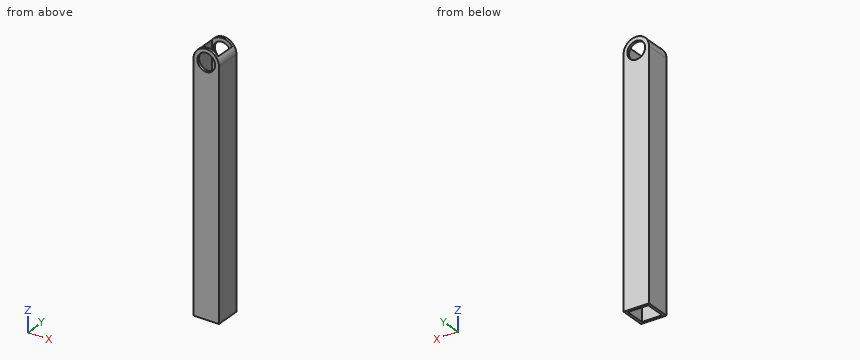
from build123d import *

# Parameters (mm, degrees)
SKETCH_1_W          = 10
SKETCH_1_H          = 10
SKETCH_1_W_2        = 8
SKETCH_1_H_2        = 8
EXTRUDE_1_DEPTH     = 100
SKETCH_2_R          = 3.5
CUT_EXTRUDE_1_DEPTH = 100


with BuildPart() as part:
    # ｽｹｯﾁ1 → ﾎﾞｽ - 押し出し1 (new body)
    with BuildSketch(Plane.XY):
        Rectangle(SKETCH_1_W, SKETCH_1_H)
        Rectangle(SKETCH_1_W_2, SKETCH_1_H_2, mode=Mode.SUBTRACT)
    extrude(amount=EXTRUDE_1_DEPTH)

    # ｽｹｯﾁ2 → ｶｯﾄ - 押し出し1 (cut)
    with BuildSketch(Plane(origin=(0, 5, 0), x_dir=(1, 0, 0), z_dir=(0, 1, 0))):
        with Locations(Location((0, -95, 0), (0, 0, 270))):
            Circle(SKETCH_2_R)
        with BuildLine():
            Line((-5, -95), (-5, -103))
            Line((-5, -103), (5, -103))
            Line((5, -103), (5, -95))
            ThreePointArc((5, -95), (0, -100), (-5, -95))
        make_face()
    extrude(amount=-CUT_EXTRUDE_1_DEPTH, mode=Mode.SUBTRACT)


solid = part.part
Could you check a few things on this model? Use its own coordinates, in mm. Round coordinates to 2 decimals unless told otherwise and drop trailing zeros. Write each loop counter-clockwise with the first axis right and the second up, starting at its lowest first coordinate (ties: lowest second). Pieces come first, ordered by that corner, then holes. Notation, with made-up numbers: (54, 74.25) - (98, 74.25) arc R31 cw to (98, 103.25) - close; hole circle Ø3 at (-35, 63.25). An arc over 180 degrees is marked (long way). Use a Markdown table: item, result.
Q1. I want a section at B-B (y = 2). List the corners of the cut face in (x, z) for me, plus the area to 3 significant figures.
Output values:
| item | result |
|---|---|
| outline | (-5, 0) - (-4, 0) - (-4, 98) arc R5 ccw to (-5, 95) - close; (4, 0) - (5, 0) - (5, 95) arc R5 ccw to (4, 98) - close |
| area | 194 mm2 |
Q2. For pin 1 (1 mm diameter, centred on x = -2, y = -0.5, fed in from +Z), with a flat end and sliding along its axis, tell me the tip position at first contact or that it passes through.
Output values:
| item | result |
|---|---|
| pin 1 | through |
Q3. I want a section at C-C (x = 1.75). List the corners of the cut face in (y, z) for me.
Output values:
| item | result |
|---|---|
| outline | (-5, 0) - (-4, 0) - (-4, 91.97) - (-5, 91.97) - close; (-5, 98.03) - (-4, 98.03) - (-4, 99.68) - (-5, 99.68) - close; (4, 0) - (5, 0) - (5, 91.97) - (4, 91.97) - close; (4, 98.03) - (5, 98.03) - (5, 99.68) - (4, 99.68) - close |
Q4. Please list where these lines run through material, in increasing order: L1, parallel to X at y = -4.7, z = 95; L2, parallel to X at y = -3, z = 87.
Output values:
| item | result |
|---|---|
| L1 | -5 to -3.5, 3.5 to 5 |
| L2 | -5 to -4, 4 to 5 |
Q5. I want a section at A-A (z = 11.5). List the corners of the cut face in (x, y) for me, plus the area to 3 significant figures.
Output values:
| item | result |
|---|---|
| outline | (-5, -5) - (5, -5) - (5, 5) - (-5, 5) - close; hole (-4, -4) - (4, -4) - (4, 4) - (-4, 4) - close |
| area | 36.0 mm2 |
